Check sheet for the modelled part. Datum: model origin and axes. Units: mm. Face numbers are marked on the shaded views. A direction names the side the tool comes from. Give positions to 0.01 mm unless a question says otherwise; leave off trailing zeros. Write each loop counter-clockwise with the first axis right and the second up, starting at its lowest first coordinate (ties: lowest second). Pieces come first, ordered by that corner, then holes. Notation, with made-up numbers: M -28.5,41.5 L -23.5,41.5 A8 cw -23.5,47.5 Z; hole C -4.75,37.5 d9. An arc over 180 degrees is marked long. Write item = value, one per line. Start each with the question number.
1) Scan lines: L1, parallel to Z at x = 13.5, y = 3.5; L2, parallel to Z at x = 4.25, y = -3; L3, parallel to X at y = -8, z = 11. Record each from-to range of solid material in increasing order.
2) Sectioned sample at D-D, the plane z = 13. Record the cut outline in (x, y).
3) Draft check along X on the marked faces 1, 2 and 3. Enter one of: pulls with the +X half, pulls with the -X half, needs draft (parallel to the pull), parting line crosses it, or undercut.
4) Sectioned sample at C-C, the plane x = 18. Record the cut outline in (y, z), then the cut area to 3 significant figures.
5) Set-up check for the marked faces 4, 5 and 6: record each of +Z, -Z, +X, -X, +Y, -Y from which the full face is reachable in a straight line by a thin tool's end or side.
6) Sectioned sample at B-B, the plane z = 8.25. Record the cut outline in (x, y), then the cut area to 3 significant figures.
7) Sectioned sample at A-A, the plane y = -18.5. Record the cut outline in (x, z), then the cut area to 3 significant figures.
8) Gauge pin test, flat ends, axial feed: pin 1 (11 mm diameter, centred on x = 10.5, y = -10, fed in from -Z); pin 2 (5 mm diameter, centred on y = -18.5, z = 7, fed in from +X); pin 3 (2 mm diameter, centred on y = -8, z = 2, fed in from +X). Record the tip position at first contact, or that the pin passes through.
from build123d import *

# Parameters (mm, degrees)
BOSS_EXTRUDE1_DEPTH      = 15.0114
SKETCH2_W                = 1.0541
SKETCH2_H                = 13.6906
CUT_EXTRUDE1_DEPTH       = 31.735742265
FILLET1_R                = 1.5
SKETCH4_W                = 0.7874
SKETCH4_H                = 7.0866
BOSS_EXTRUDE2_DEPTH      = 12.9032
SKETCH5_W                = 4.0767
SKETCH5_H                = 7.0866
CUT_EXTRUDE2_DEPTH       = 34.156380129
BOSS_EXTRUDE3_DEPTH      = 4
BOSS_EXTRUDE3_DEPTH_BACK = 4


with BuildPart() as part:
    # Sketch1 → Boss-Extrude1 (new body)
    with BuildSketch(Plane.XY):
        Polygon((-2.032, 0), (0, 0), (0, -13.6906), (18.9992, -13.6906), (18.9992, 0), (21.0312, 0), (21.0312, 2.0066), (-2.032, 2.0066), align=None)
    extrude(amount=BOSS_EXTRUDE1_DEPTH)

    # Sketch2 → Cut-Extrude1 (cut, through all)
    with BuildSketch(Plane(origin=(21.0312, 0, 0), x_dir=(0, 0, -1), z_dir=(1, 0, 0))):
        with Locations((-14.48435, -6.8453)):
            Rectangle(SKETCH2_W, SKETCH2_H)
        with Locations((-0.52705, -6.8453)):
            Rectangle(SKETCH2_W, SKETCH2_H)
    extrude(amount=-CUT_EXTRUDE1_DEPTH, mode=Mode.SUBTRACT)

    # Fillet1
    fillet1_edges = [part.edges().sort_by_distance(p)[0] for p in [
        (-2.032, 2.0066, 7.5057),
        (21.0312, 2.0066, 7.5057),
        (9.4996, 2.0066, 15.0114),
        (9.4996, 2.0066, 0),
    ]]
    fillet(fillet1_edges, radius=FILLET1_R)

    # Sketch4 → Boss-Extrude2 (add)
    with BuildSketch(Plane.XY.offset(13.9573)):
        with Locations((2.5146, -17.2339)):
            Rectangle(SKETCH4_W, SKETCH4_H)
        with Locations((9.4996, -17.2339)):
            Rectangle(SKETCH4_W, SKETCH4_H)
    extrude(amount=-BOSS_EXTRUDE2_DEPTH)

    # Sketch5 → Cut-Extrude2 (cut, through all)
    with BuildSketch(Plane.ZY):
        with Locations((3.09245, -17.2339)):
            Rectangle(SKETCH5_W, SKETCH5_H)
        with Locations((11.91895, -17.2339)):
            Rectangle(SKETCH5_W, SKETCH5_H)
    extrude(amount=-CUT_EXTRUDE2_DEPTH, mode=Mode.SUBTRACT)

    # Sketch6 → Boss-Extrude3 (add, two sides: drawn at the far end of the back side and taken through both)
    with BuildSketch(Plane.XY.offset(7.5057).offset(-BOSS_EXTRUDE3_DEPTH_BACK)):
        with BuildLine():
            Line((2.163304729, 4.48357977), (1.4996, 2.0066))
            Line((1.4996, 2.0066), (17.4996, 2.0066))
            Line((17.4996, 2.0066), (16.835895271, 4.48357977))
            ThreePointArc((16.835895271, 4.48357977), (16.571901131, 4.803672947), (16.157122862, 4.814233984))
            ThreePointArc((16.157122862, 4.814233984), (9.4996, 3.456401012), (2.842077138, 4.814233984))
            ThreePointArc((2.842077138, 4.814233984), (2.427298869, 4.803672947), (2.163304729, 4.48357977))
        make_face()
    extrude(amount=BOSS_EXTRUDE3_DEPTH + BOSS_EXTRUDE3_DEPTH_BACK)


solid = part.part
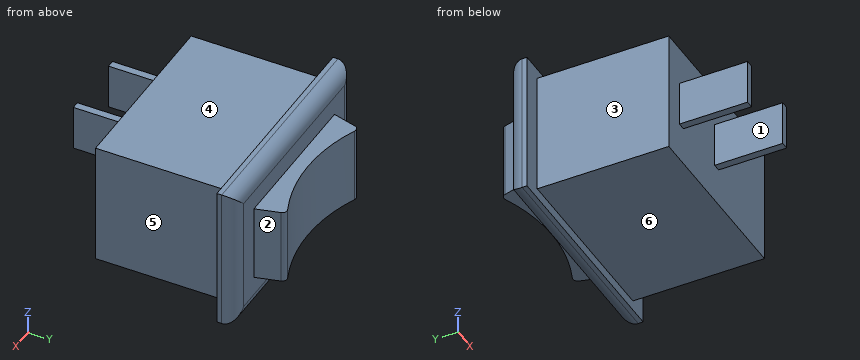
Data:
q1.L1 = 3.51 to 11.51
q1.L2 = 1.05 to 13.96
q1.L3 = 0 to 19
q2.outline = M -2.03,0 L 0,0 L 0,-13.69 L 19,-13.69 L 19,0 L 21.03,0 L 21.03,0.51 A1.5 ccw 19.53,2.01 L -0.53,2.01 A1.5 ccw -2.03,0.51 Z
q3.face_1 = undercut
q3.face_2 = pulls with the +X half
q3.face_3 = pulls with the -X half
q4.outline = M -13.69,1.05 L 0,1.05 L 0,0 L 0.51,0 A1.5 ccw 2.01,1.5 L 2.01,13.51 A1.5 ccw 0.51,15.01 L 0,15.01 L 0,13.96 L -13.69,13.96 Z
q4.area = 206 mm2
q5.face_4 = +Z, +X, -X, -Y
q5.face_5 = +Z, -Z, +X, -Y
q5.face_6 = -Z, +X, -X, -Y
q6.outline = M -2.03,0 L 0,0 L 0,-13.69 L 2.12,-13.69 L 2.12,-20.78 L 2.91,-20.78 L 2.91,-13.69 L 9.11,-13.69 L 9.11,-20.78 L 9.89,-20.78 L 9.89,-13.69 L 19,-13.69 L 19,0 L 21.03,0 L 21.03,0.51 A1.5 ccw 19.53,2.01 L 17.5,2.01 L 16.84,4.48 A0.5 ccw 16.16,4.81 A17 cw 2.84,4.81 A0.5 ccw 2.16,4.48 L 1.5,2.01 L -0.53,2.01 A1.5 ccw -2.03,0.51 Z
q6.area = 347 mm2
q7.outline = M 2.12,5.13 L 2.91,5.13 L 2.91,9.88 L 2.12,9.88 Z; M 9.11,5.13 L 9.89,5.13 L 9.89,9.88 L 9.11,9.88 Z
q7.area = 7.48 mm2
q8.pin_1 = 1.05
q8.pin_2 = 9.89
q8.pin_3 = 19
